The listing builds one solid part. Answer for the finished solid, in the listing's coordinates (mm). Face numbers are marked on the shaded views. A direction names the side the tool comes from. Give positions to 0.01 mm unless a question says otherwise; leave off trailing zeros. Loops run counter-clockwise (first coordinate to the right, second up) from the corner with the lowest first, then second, coordinate; pieces in that order, holes last. Notation, with made-up numbers: (-36, 72.25) - (-25, 72.25) arc R19 ccw to (-25, 109.25) - close; hole circle Ø10 at (-22, 83). An arc over 180 degrees is marked (long way). One line per item, written item: value. Start each with the question number.
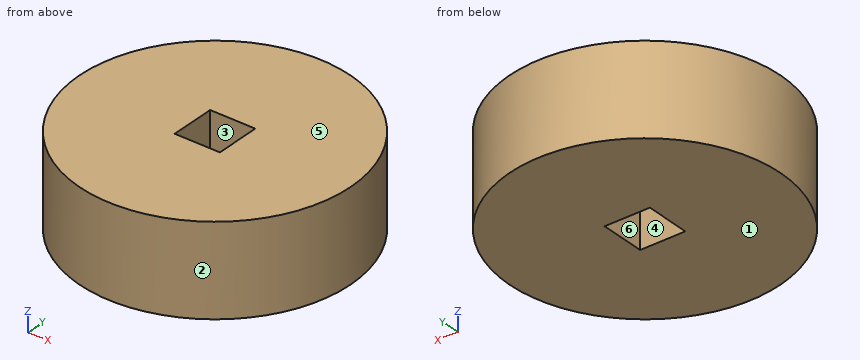
Autodesk Inventor part; units mm, degrees
ref_plane "YZ Plane" through (0, 0, 0) normal (1, 0, 0) x (0, 1, 0)
ref_plane "XZ Plane" through (0, 0, 0) normal (0, 1, 0) x (-1, 0, 0)
ref_plane "XY Plane" through (0, 0, 0) normal (0, 0, 1) x (1, 0, 0)
sketch "Sketch1" plane through (0, 0, 0) normal (0, 0, 1) x (1, 0, 0)
  circle A0 centre (0, 0) radius 38.1
  line L0 (-6.35, 6.35) -> (6.35, 6.35)
  line L1 (6.35, 6.35) -> (6.35, -6.35)
  line L2 (6.35, -6.35) -> (-6.35, -6.35)
  line L3 (-6.35, -6.35) -> (-6.35, 6.35)
  dimension "d0" = 76.2
  dimension "d1" = 12.7
  dimension "d2" = 12.7
  dimension "d3" = 6.35
  dimension "d4" = 6.35
extrude "Extrusion1" add sketch "Sketch1" along normal blind 25.4
properties part number "Random Compliance Wheel"
1. For the marked faces 5 and 6, determine the directions among +Z, -Z, +X, -X, +Y, -Y from which every point of the face is accessible in a straight line to the end or side of a thin tool.
2. A cutting plane is placed at A-A (x = 0). Determine the outline of the cut face in (y, z).
3. Determine the mould class of the marked faces 1, 2, 3 and 4 for opening direction Y: released by +Y, released by -Y, zero draft, split by the parting line, or undercut.
4. Flat-ended cylindrical pins translate along their axes: pin 1 (8 mm diameter, centred on x = -21.5, z = 9, fed in from -Y); pin 2 (1 mm diameter, centred on y = 16.5, z = 15.5, fed in from +X); pin 3 (6.5 mm diameter, centred on x = -3, z = 9.5, fed in from -Y). Find the tip coordinate at first contact, or state that the pin passes through.
5. Find the intervals of material crossed by L1, parallel to Y at x = -1, z = 11.75; L2, parallel to Y at x = 2.5, z = 9.25, in increasing order. Write a range as [from, to].
6. A cutting plane is placed at D-D (x = -28). Determine the outline of the cut face in (y, z).
7. A cutting plane is placed at C-C (z = 23). Determine the outline of the cut face in (x, y), plus the area to 3 significant figures.
Results below:
1. face 5: +Z, +X, -X, +Y, -Y
1. face 6: +Z, -Z
2. outline: (-38.1, 0) - (-6.35, 0) - (-6.35, 25.4) - (-38.1, 25.4) - close; (6.35, 0) - (38.1, 0) - (38.1, 25.4) - (6.35, 25.4) - close
3. face 1: zero draft
3. face 2: split by the parting line
3. face 3: undercut
3. face 4: undercut
4. pin 1: stops at y = -33.84
4. pin 2: stops at x = 34.58
4. pin 3: stops at y = -38.1
5. L1: y = [-38.09, -6.35], [6.35, 38.09]
5. L2: y = [-38.02, -6.35], [6.35, 38.02]
6. outline: (-25.84, 0) - (25.84, 0) - (25.84, 25.4) - (-25.84, 25.4) - close
7. outline: circle Ø76.2 at (0, 0); hole (-6.35, -6.35) - (6.35, -6.35) - (6.35, 6.35) - (-6.35, 6.35) - close
7. area: 4,400 mm^2
